from build123d import *

# Parameters (mm, degrees)
SKETCH3_W              = 75
SKETCH3_H              = 300
BOSS_EXTRUDE1_DEPTH    = 15
SKETCH4_R              = 20
CUT_EXTRUDE1_DEPTH     = 5
FILLET1_R              = 5
BOSS_EXTRUDE4_DEPTH    = 65
FILLET3_R              = 10
FILLET4_R              = 10
SKETCH12_W             = 50
SKETCH12_H             = 20
BOSS_EXTRUDE5_DEPTH    = 4
FILLET5_R              = 10
LPATTERN3_COUNT        = 7
LPATTERN3_PITCH        = 25
FILLET5_OF_LPATTERN3_R = 10


with BuildPart() as part:
    # Sketch3 → Boss-Extrude1 (new body)
    with BuildSketch(Plane.XY):
        Rectangle(SKETCH3_W, SKETCH3_H)
    extrude(amount=BOSS_EXTRUDE1_DEPTH)

    # Sketch4 → Cut-Extrude1 (cut)
    with BuildSketch(Plane(origin=(0, 0, 0), x_dir=(-1, 0, 0), z_dir=(0, 0, -1))):
        with Locations((0, -120)):
            Circle(SKETCH4_R)
    extrude(amount=-CUT_EXTRUDE1_DEPTH, mode=Mode.SUBTRACT)

    # Fillet1
    fillet1_edges = [part.edges().sort_by_distance(p)[0] for p in [
        (37.5, 0, 15),
        (-37.5, 0, 15),
        (37.5, 0, 0),
        (-37.5, 0, 0),
    ]]
    fillet(fillet1_edges, radius=FILLET1_R)

    # Sketch11 → Boss-Extrude4 (add)
    with BuildSketch(Plane(origin=(32.5, 0, 0), x_dir=(0, 0, -1), z_dir=(1, 0, 0))):
        with BuildLine():
            Line((-15, 150), (-15, -55.184099518))
            add(Edge.make_bspline(
                [(-15, -55.184099518), (-36.150035241, -75.256670259), (-50.395734878, -100.703118223)],
                knots=[0, 0, 0, 1, 1, 1], degree=2))
            Line((-50.395734878, -100.703118223), (-50.395734878, 150))
            Line((-50.395734878, 150), (-15, 150))
        make_face()
    extrude(amount=-BOSS_EXTRUDE4_DEPTH)

    # Fillet3
    fillet3_edges = [part.edges().sort_by_distance(p)[0] for p in [
        (-32.5, 24.648440888, 50.395734878),
    ]]
    fillet(fillet3_edges, radius=FILLET3_R)

    # Fillet4
    fillet4_edges = [part.edges().sort_by_distance(p)[0] for p in [
        (32.5, 24.648440888, 50.395734878),
    ]]
    fillet(fillet4_edges, radius=FILLET4_R)

    # Sketch12 → Boss-Extrude5 (add)
    with BuildSketch(Plane(origin=(0, 0, 0), x_dir=(-1, 0, 0), z_dir=(0, 0, -1))):
        with Locations((-1.606045565, -56.843050926)):
            Rectangle(SKETCH12_W, SKETCH12_H)
    boss_extrude5 = extrude(amount=BOSS_EXTRUDE5_DEPTH)

    # Fillet5
    fillet5_edges = [part.edges().sort_by_distance(p)[0] for p in [
        (-23.393954435, -66.843050926, -2),
        (-23.393954435, -46.843050926, -2),
        (26.606045565, -66.843050926, -2),
        (26.606045565, -46.843050926, -2),
    ]]
    fillet(fillet5_edges, radius=FILLET5_R - 0.0001)  # a hair under: the kernel refuses the full size

    # LPattern3: Boss-Extrude5 ×7
    with Locations(*[(0, i * LPATTERN3_PITCH, 0) for i in range(1, LPATTERN3_COUNT)]):
        add(boss_extrude5)

    # Fillet5 of LPattern3
    fillet5_of_lpattern3_edges = [part.edges().sort_by_distance(p)[0] for p in [
        (-23.393954435, -41.843050926, -2),
        (-23.393954435, -21.843050926, -2),
        (26.606045565, -41.843050926, -2),
        (26.606045565, -21.843050926, -2),
        (-23.393954435, -16.843050926, -2),
        (-23.393954435, 3.156949074, -2),
        (26.606045565, -16.843050926, -2),
        (26.606045565, 3.156949074, -2),
        (-23.393954435, 8.156949074, -2),
        (-23.393954435, 28.156949074, -2),
        (26.606045565, 8.156949074, -2),
        (26.606045565, 28.156949074, -2),
        (-23.393954435, 33.156949074, -2),
        (-23.393954435, 53.156949074, -2),
        (26.606045565, 33.156949074, -2),
        (26.606045565, 53.156949074, -2),
        (-23.393954435, 58.156949074, -2),
        (-23.393954435, 78.156949074, -2),
        (26.606045565, 58.156949074, -2),
        (26.606045565, 78.156949074, -2),
        (-23.393954435, 83.156949074, -2),
        (-23.393954435, 103.156949074, -2),
        (26.606045565, 83.156949074, -2),
        (26.606045565, 103.156949074, -2),
    ]]
    fillet(fillet5_of_lpattern3_edges, radius=FILLET5_OF_LPATTERN3_R - 0.0001)  # a hair under: the kernel refuses the full size


solid = part.part
Here's how the part is built. I have some questions about the finished solid (model axes, mm). A direction names the side the tool comes from. Round coordinates to 2 decimals unless told otherwise and drop trailing zeros. Write each loop counter-clockwise with the first axis right and the second up, starting at its lowest first coordinate (ties: lowest second). Pieces come first, ordered by that corner, then holes.
1. If we mould it in two halves opening along Y, with no side actions, what happens to faces 5 (the cylindrical face through (29.493, 26.403, 47.544)), 6 (the cylindrical face through (23.754, -49.85, -2.028)), 7 (the flat face through (1, 150, 26)), 8 (the cylindrical face through (-20.387, 75.305, -2.028))? For each: released by +Y, released by -Y, zero draft, split by the parting line, or undercut.
2. For faces 1 (the flat face through (0, -102, 15)), 2 (the cylindrical face through (-20.54, -38.84, -2.03)), 3 (the cylindrical face through (23.754, 50.15, -2.028)), 4 (the flat face through (0, -120, 5)), which set-ups out of +Z, -Z, +X, -X, +Y, -Y let a thin tool reach every point of the face, with its end or its side?
3. Suppose I cut it at B-B (y = 131). List the corners of the cut face in (x, z) for me, and give its area (3 significant figures).
4. Will these pins go through, and if not, where does the flat tip stop? pin 1 Ø1.2 at (x, z) = (-4.5, -2.5) entering from -Y; pin 2 Ø2 at (x, z) = (4.5, -1.5) entering from +Y; pin 3 Ø4 at (y, z) = (94.5, 32) entering from -X.
5. Suppose I cut it at A-A (y = -120). List the corners of the cut face in (x, z) for me.
6. I need wall thicknesses on L1, parallel to Y at x = 0, z = 1.55; L2, parallel to Z at x = -4, y = -113; L3, parallel to X at y = -8.5, z = 24.5. Which ranges of each line are inside material? Lowest first, please.
Answer sheet:
1. face 5: zero draft
1. face 6: undercut
1. face 7: released by +Y
1. face 8: undercut
2. face 1: +X, -X, -Y
2. face 2: -Z, -X
2. face 3: -Z, +X
2. face 4: -Z
3. outline: (-37.5, 5) arc R5 ccw to (-32.5, 0) - (32.5, 0) arc R5 ccw to (37.5, 5) - (37.5, 10) arc R5 ccw to (32.5, 15) - (32.5, 40.4) arc R10 ccw to (22.5, 50.4) - (-22.5, 50.4) arc R10 ccw to (-32.5, 40.4) - (-32.5, 15) arc R5 ccw to (-37.5, 10) - close
3. area: 3,360 mm2
4. pin 1: stops at y = -66.84
4. pin 2: stops at y = 103.16
4. pin 3: stops at x = -32.5
5. outline: (-37.5, 5) arc R5 ccw to (-32.5, 0) - (-20, 0) - (-20, 5) - (20, 5) - (20, 0) - (32.5, 0) arc R5 ccw to (37.5, 5) - (37.5, 10) arc R5 ccw to (32.5, 15) - (-32.5, 15) arc R5 ccw to (-37.5, 10) - close
6. L1: y = -150 to -140, -100 to 150
6. L2: z = 5 to 15
6. L3: x = -32.5 to 32.5
